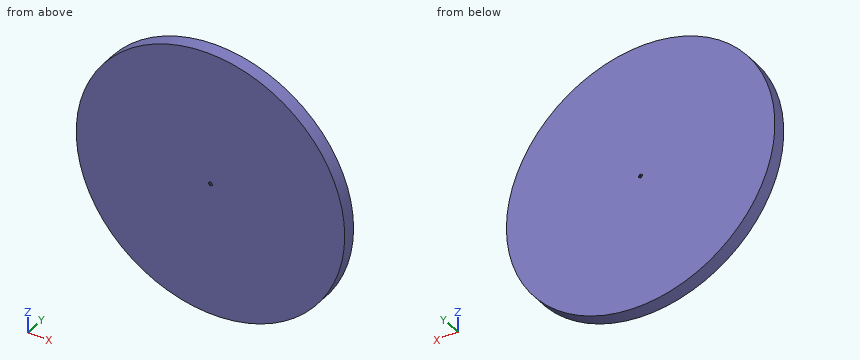
from build123d import *

# Parameters (mm, degrees)
SKETCH1_R           = 50
BOSS_EXTRUDE1_DEPTH = 5


with BuildPart() as part:
    # Sketch1 → Boss-Extrude1 (new body)
    with BuildSketch(Plane(origin=(0, 0, 0), x_dir=(1, 0, 0), z_dir=(0, 1, 0))):
        Circle(SKETCH1_R)
        Polygon((0.012163769, -0.721880139), (-0.338076022, -0.721880139), (-0.338076022, -0.338076022), (-0.721880139, -0.338076022), (-0.721880139, -0.012163769), (-0.721880139, 0.012163769), (-0.721880139, 0.338076022), (-0.338076022, 0.338076022), (-0.338076022, 0.721880139), (0.012163769, 0.721880139), (0.362204732, 0.710080322), (0.34927411, 0.326494088), (0.732860345, 0.313563466), (0.722290178, 0), (0.732860345, -0.313563466), (0.34927411, -0.326494088), (0.362204732, -0.710080322), align=None, mode=Mode.SUBTRACT)
    extrude(amount=BOSS_EXTRUDE1_DEPTH)


solid = part.part
CAD build for the part. Positions are in the model's coordinates, mm. Give positions to 0.01 mm unless a question says otherwise; leave off trailing zeros. Loops run counter-clockwise (first coordinate to the right, second up) from the corner with the lowest first, then second, coordinate; pieces in that order, holes last. Notation, with made-up numbers: M 51.25,34.25 L 86.25,34.25 A8 cw 86.25,47.25 Z; hole C -15,10.25 d9. An arc over 180 degrees is marked long. Write each question's results on one line, items separated by ' | '.
Q1. Band-saw the part on B-B on z = 25.5. Write the cut outline in (x, y).
Geometry check:
outline: M -43.01,0 L 43.01,0 L 43.01,5 L -43.01,5 Z
Q2. Probe probe 1 along Z at (x, y) = (-1, 4.5); probe 2 along Z at (x, y) = (38, 1.45); probe 3 along X at (y, z) = (2, -18.5). List the from-to ranges inside material, lowest first.
Geometry check:
probe 1: z = -49.99 to 49.99 | probe 2: z = -32.5 to 32.5 | probe 3: x = -46.45 to 46.45
Q3. Band-saw the part on C-C on x = -44. Write the cut outline in (y, z), and give its area (3 significant figures).
Geometry check:
outline: M 0,-23.75 L 5,-23.75 L 5,23.75 L 0,23.75 Z | area: 237 mm²
Q4. Band-saw the part on A-A on y = 0.95. Write the cut outline in (x, z), and give its area (3 significant figures).
Geometry check:
outline: C 0,0 d100; hole M -0.72,-0.34 L -0.34,-0.34 L -0.34,-0.72 L 0.01,-0.72 L 0.36,-0.71 L 0.35,-0.33 L 0.73,-0.31 L 0.72,0 L 0.73,0.31 L 0.35,0.33 L 0.36,0.71 L 0.01,0.72 L -0.34,0.72 L -0.34,0.34 L -0.72,0.34 Z | area: 7,850 mm²
Q5. Flat gauge pins, fed straight in: P1, Ø1.5, axis at x = -9.5, y = 2, coming from the +Z side; P2, Ø1, axis at x = -32.5, y = 4, coming from the +Z side. Where does each tip first touch, or does it go through?
Geometry check:
P1: stops at z = 49.23 | P2: stops at z = 38.42
